Autodesk Inventor part; units mm, degrees
ref_plane "YZ Plane" through (0, 0, 0) normal (1, 0, 0) x (0, 1, 0)
ref_plane "XZ Plane" through (0, 0, 0) normal (0, 1, 0) x (-1, 0, 0)
ref_plane "XY Plane" through (0, 0, 0) normal (0, 0, 1) x (1, 0, 0)
sketch "Skizze1" plane through (0, 0, 0) normal (0, 0, 1) x (1, 0, 0)
  circle A0 centre (0, 0) radius 3.1
  circle A1 centre (0, 0) radius 4.6
  circle A2 centre (0, 0) radius 2.1
  dimension "d0" = 6.2
  dimension "d1" = 1.5
  dimension "d2" = 4.2
extrude "Extrusion1" add sketch "Skizze1" against normal blind 4 contours A0 | A1
extrude "Extrusion2" add sketch "Skizze1" along normal blind 2 contours A1
properties part number "MagnetHolder"
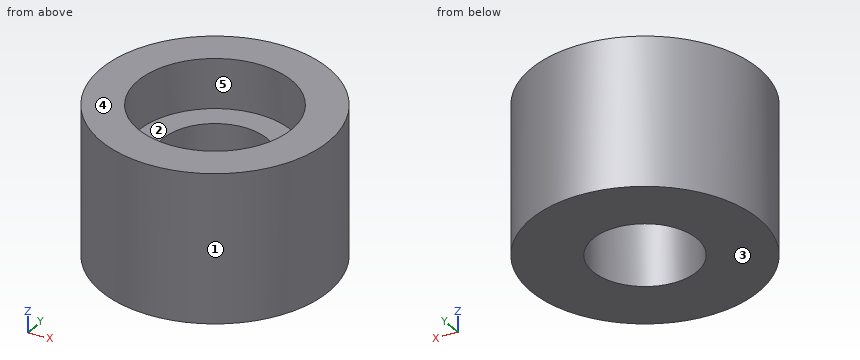
Design review of the part built by this model. Coordinates are the model's own, in mm. Face numbers are marked on the shaded views. A direction names the side the tool comes from. Give positions to 0.01 mm unless a question says otherwise; leave off trailing zeros. Write each loop counter-clockwise with the first axis right and the second up, starting at its lowest first coordinate (ties: lowest second). Pieces come first, ordered by that corner, then holes. Notation, with made-up numbers: (12, -2.5) - (30, -2.5) arc R19 ccw to (30, 5.5) - close; hole circle Ø1 at (-38, -2). An arc over 180 degrees is marked (long way). Return JSON: item names as keys, results as strings. Group by question number.
(1) Machinability: for the marked faces 4 and 5, which of the approach directions +Z, -Z, +X, -X, +Y, -Y give a long, thin tool a straight path to every point of the face, cutting with its end or side? Answer none if there is none.
(2) To check wall thickness, follow probe 1 along Y at (x, z) = (0, -1.6); probe 2 along Y at (x, z) = (0, 1.25); probe 3 along Z at (x, y) = (2, -0.75). State the ranges of each line that lie inside material, in increasing order.
(3) Insertion check: pin 1 (3 mm diameter, centred on x = 2, z = -1, fed in from -Y). The pin has a flat end and moves straight along its axis. Give the tip position at first contact, or say it passes through.
(4) Mouldability with a two-part tool opening along Y and no side actions: class the marked faces 1, 2 and 3 as +Y half, -Y half, draft (parallel to the pull), parting line (faces both ways), or undercut.
(5) We need section D-D, the plane x = -2.25. Give the boundary of the cut face in (y, z).
(6) We need section A-A, the plane x = 0. Give the boundary of the cut face in (y, z).
(7) We need section C-C, the plane z = 0.75. Give the boundary of the cut face in (x, y), then the cut area to 3 significant figures.
Reported:
{
 "1": {"face 4": "+Z, +X, -X, +Y, -Y", "face 5": "+Z"},
 "2": {"probe 1": "y = -4.6 to -2.1, 2.1 to 4.6", "probe 2": "y = -4.6 to -3.1, 3.1 to 4.6", "probe 3": "z = -4 to 0"},
 "3": {"pin 1": "stops at y = -4.57"},
 "4": {"face 1": "parting line", "face 2": "undercut", "face 3": "draft"},
 "5": {"outline": "(-4.01, -4) - (4.01, -4) - (4.01, 2) - (2.13, 2) - (2.13, 0) - (-2.13, 0) - (-2.13, 2) - (-4.01, 2) - close"},
 "6": {"outline": "(-4.6, -4) - (-2.1, -4) - (-2.1, 0) - (-3.1, 0) - (-3.1, 2) - (-4.6, 2) - close; (2.1, -4) - (4.6, -4) - (4.6, 2) - (3.1, 2) - (3.1, 0) - (2.1, 0) - close"},
 "7": {"outline": "circle Ø9.2 at (0, 0); hole circle Ø6.2 at (0, 0)", "area": "36.3 mm2"}
}
